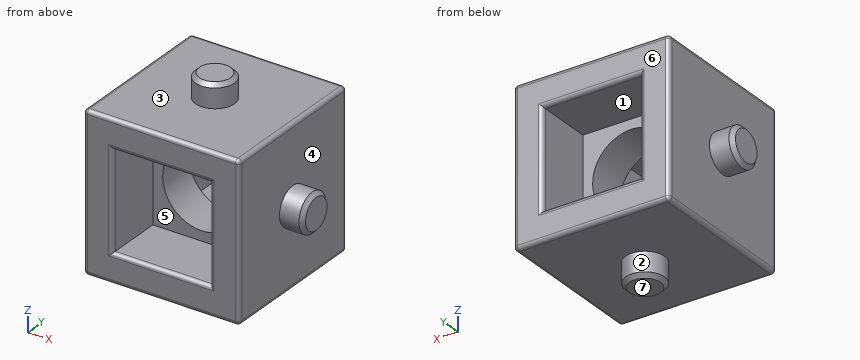
```python
from build123d import *

# Parameters (mm, degrees)
SKETCH_1_W          = 8
SKETCH_1_H          = 8
EXTRUDE_1_DEPTH     = 8
SKETCH_2_W          = 5
SKETCH_2_H          = 5
CUT_EXTRUDE_1_DEPTH = 3
SKETCH_3_W          = 5
SKETCH_3_H          = 5
CUT_EXTRUDE_2_DEPTH = 3
CUT_EXTRUDE_3_REACH = 9.55
SKETCH_4_R          = 2
SKETCH_5_R          = 1
EXTRUDE_2_DEPTH     = 1.2
SKETCH_6_R          = 1
EXTRUDE_3_DEPTH     = 1.2
CHAMFER_1_SIZE      = 0.2
FILLET_1_R          = 0.2


with BuildPart() as part:
    # 草图1 → 凸台-拉伸1 (new body)
    with BuildSketch(Plane(origin=(0, 0, 0), x_dir=(1, 0, 0), z_dir=(0, 1, 0))):
        Rectangle(SKETCH_1_W, SKETCH_1_H)
    extrude(amount=EXTRUDE_1_DEPTH)

    # 草图2 → 切除-拉伸1 (cut)
    with BuildSketch(Plane(origin=(0, 8, 0), x_dir=(1, 0, 0), z_dir=(0, 1, 0))):
        Rectangle(SKETCH_2_W, SKETCH_2_H)
    extrude(amount=-CUT_EXTRUDE_1_DEPTH, mode=Mode.SUBTRACT)

    # 草图3 → 切除-拉伸2 (cut)
    with BuildSketch(Plane.XZ):
        Rectangle(SKETCH_3_W, SKETCH_3_H)
    extrude(amount=-CUT_EXTRUDE_2_DEPTH, mode=Mode.SUBTRACT)

    # 草图4 → 切除-拉伸3 (cut, up to next)
    with BuildSketch(Plane.XZ.offset(-3), mode=Mode.PRIVATE) as cut_extrude_3_sk1:
        with Locations(Location((0, 0, 0), (0, 0, 270))):
            Circle(SKETCH_4_R)
    cut_extrude_3_tool1 = extrude(cut_extrude_3_sk1.sketch, amount=-CUT_EXTRUDE_3_REACH, mode=Mode.PRIVATE) & part.part
    add(cut_extrude_3_tool1.solids().sort_by_distance((0, 3, 0))[0], mode=Mode.SUBTRACT)

    # 草图5 → 凸台-拉伸2 (add)
    with BuildSketch(Plane.ZY.offset(4)):
        with Locations(Location((0, 4, 0), (0, 0, 180))):
            Circle(SKETCH_5_R)
    extrude_2 = extrude(amount=EXTRUDE_2_DEPTH)

    # 镜向1: 凸台-拉伸2 across plane
    add(extrude_2.mirror(Plane(origin=(0, 0, 0), x_dir=(0, 0, 1), z_dir=(1, 0, 0))))

    # 草图6 → 凸台-拉伸3 (add)
    with BuildSketch(Plane(origin=(0, 0, -4), x_dir=(-1, 0, 0), z_dir=(0, 0, -1))):
        with Locations(Location((0, 4, 0), (0, 0, 180))):
            Circle(SKETCH_6_R)
    extrude_3 = extrude(amount=EXTRUDE_3_DEPTH)

    # 镜向2: 凸台-拉伸3 across plane
    add(extrude_3.mirror(Plane.XY))

    # 倒角1
    chamfer_1_edges = [part.edges().sort_by_distance(p)[0] for p in [
        (-5.2, 4, 1),
        (5.2, 4, 1),
        (-1, 4, -5.2),
        (-1, 4, 5.2),
    ]]
    chamfer(chamfer_1_edges, length=CHAMFER_1_SIZE)

    # 圆角1
    fillet_1_edges = [part.edges().sort_by_distance(p)[0] for p in [
        (0, 8, 4),
        (4, 8, 0),
        (2.5, 8, 0),
        (0, 8, -2.5),
        (-2.5, 8, 0),
        (0, 8, 2.5),
        (-2.5, 0, 0),
        (0, 0, -2.5),
        (2.5, 0, 0),
        (0, 0, 2.5),
        (0, 8, -4),
        (4, 0, 0),
        (0, 0, 4),
        (-4, 0, 0),
        (0, 0, -4),
        (-4, 8, 0),
        (4, 4, -4),
        (4, 4, 4),
        (-4, 4, 4),
        (-4, 4, -4),
    ]]
    fillet(fillet_1_edges, radius=FILLET_1_R)


solid = part.part
```
Geometry check sheet. Reference: the model listing, model coordinates, mm. Face numbers are marked on the shaded views. A direction names the side the tool comes from. Give positions to 0.01 mm unless a question says otherwise; leave off trailing zeros. Order: outer loops, then holes, each group sorted by start corner. A loop starts at its lowest first (then second) coordinate and runs counter-clockwise, first axis right, second up. Notation, with made-up numbers: (73, 48.5) - (108, 48.5) arc R19 cw to (108, 83.5) - close; hole circle Ø11 at (77.25, 53). An arc over 180 degrees is marked (long way). Write item = value, one per line. Start each with the question number.
1) Gauge pin test, flat ends, axial feed: pin 1 Ø0.8 at (y, z) = (1.5, -1) entering from -X; pin 2 Ø0.8 at (x, y) = (-0.5, 2) entering from +Z; pin 3 Ø0.8 at (x, y) = (1, 6) entering from -Z; pin 4 Ø3.5 at (x, z) = (0, 0) entering from -Y. Record the tip position at first contact, or that the pin passes through.
2) Section check B-B (z = -3.25). Enter the section's corners in (x, y), then the cut area to 3 significant figures.
3) Access from +Z, -Z, +X, -X, +Y, -Y to the whole of each face (thin tool, end or side, straight path). Record for the marked faces 1, 2, 3 and 4.
4) Draft check along Z on the marked faces 5, 6 and 7. Enter one of: released by +Z, released by -Z, zero draft, split by the parting line, or undercut.
5) Section check C-C (y = 2.5). Enter the section's corners in (x, z).
6) Scan lines: L1, parallel to X at y = 4.55, z = 0; L2, parallel to Z at x = -2, y = 0.5; L3, parallel to Y at x = -2.25, z = 2. Record each from-to range of solid material in increasing order.
Geometry check:
q1.pin_1 = -4
q1.pin_2 = 4
q1.pin_3 = -4
q1.pin_4 = through
q2.outline = (-4, 0.2) arc R0.2 ccw to (-3.8, 0) - (3.8, 0) arc R0.2 ccw to (4, 0.2) - (4, 7.8) arc R0.2 ccw to (3.8, 8) - (-3.8, 8) arc R0.2 ccw to (-4, 7.8) - close
q2.area = 64.0 mm2
q3.face_1 = +Y
q3.face_2 = -Z
q3.face_3 = +Z
q3.face_4 = +X
q4.face_5 = undercut
q4.face_6 = zero draft
q4.face_7 = released by -Z
q5.outline = (-4, -3.8) arc R0.2 ccw to (-3.8, -4) - (3.8, -4) arc R0.2 ccw to (4, -3.8) - (4, 3.8) arc R0.2 ccw to (3.8, 4) - (-3.8, 4) arc R0.2 ccw to (-4, 3.8) - close; hole (-2.5, -2.5) - (2.5, -2.5) - (2.5, 2.5) - (-2.5, 2.5) - close
q6.L1 = -5.2 to -2, 2 to 5.2
q6.L2 = -4 to -2.5, 2.5 to 4
q6.L3 = 3 to 5
